Part model, mm, in its own coordinate system. Face numbers are marked on the shaded views. Round coordinates to 2 decimals unless told otherwise and drop trailing zeros. Loops run counter-clockwise (first coordinate to the right, second up) from the corner with the lowest first, then second, coordinate; pieces in that order, holes last. Notation, with made-up numbers: M -32.75,-13 L -15.75,-13 A32 cw -15.75,14 Z; hole C 62,63 d11. An arc over 180 degrees is marked long. Put each result on its own line as item: value. Start each with the question number.
1) Slice it at C-C on z = 5. Give the cut face in (x, y).
2) Probe line 1 along X through (y, z) = (21, 60); line 2 along X through (y, z) = (19, 41); line 3 along Y through (x, z) = (21, 47). List the from-to ranges inside material, lowest first.
3) Pull direction Y, two halves, no side cores. Call the marked faces 1, 2 and 3: +Y half, -Y half, draft (parallel to the pull), parting line (faces both ways), or undercut.
4) Drop flat-ended pins along their axis: pin 1 Ø1.1 at (x, y) = (2.5, 2) entering from -Z; pin 2 Ø8 at (x, z) = (27.5, 37) entering from -Y; pin 3 Ø2 at (x, z) = (21.5, 46.5) entering from +Y; pin 4 Ø0.8 at (x, z) = (30.5, 89.5) entering from -Y. Give the stop position or say it passes through.
5) Slice it at A-A on y = 5. Give the cut face in (x, z).
6) Slice it at B-B on z = 50. Give the cut face in (x, y), then the cut area to 3 significant figures.
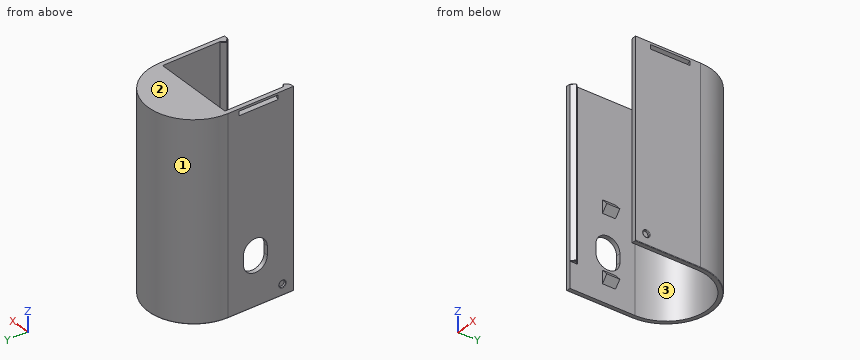
```python
from build123d import *

# Parameters (mm, degrees)
BOSS_EXTRUDE1_DEPTH = 90
BOSS_EXTRUDE2_START = -1
BOSS_EXTRUDE2_DEPTH = 1
CUT_EXTRUDE2_DEPTH  = 2
SKETCH6_R           = 1.5
CUT_EXTRUDE3_DEPTH  = 1
CUT_EXTRUDE4_DEPTH  = 18
BOSS_EXTRUDE3_DEPTH = 78
BOSS_EXTRUDE4_START = -8
BOSS_EXTRUDE4_DEPTH = 6
FILLET2_R           = 0.25
CHAMFER1_SIZE       = 0.25
FILLET3_R           = 0.25
CHAMFER2_SIZE       = 0.25


with BuildPart() as part:
    # Sketch2 → Boss-Extrude1 (new body)
    with BuildSketch(Plane.XY):
        with BuildLine():
            Line((0, 0), (0, 30))
            ThreePointArc((0, 30), (21, 51), (42, 30))
            Line((42, 30), (42, 0))
            Line((42, 0), (40, 0))
            Line((40, 0), (40, 30))
            ThreePointArc((40, 30), (21, 49), (2, 30))
            Line((2, 30), (2, 0))
            Line((2, 0), (0, 0))
        make_face()
    extrude(amount=BOSS_EXTRUDE1_DEPTH)

    # Sketch3 → Boss-Extrude2 (add)
    with BuildSketch(Plane.XY.offset(90).offset(BOSS_EXTRUDE2_START)):
        with BuildLine():
            Line((2, 30), (40, 30))
            ThreePointArc((40, 30), (21, 49), (2, 30))
        make_face()
    extrude(amount=BOSS_EXTRUDE2_DEPTH)

    # Sketch5 → Cut-Extrude2 (cut)
    with BuildSketch(Plane.ZY):
        with BuildLine():
            Line((20.5, 23), (24.5, 23))
            ThreePointArc((24.5, 23), (30, 17.5), (24.5, 12))
            Line((24.5, 12), (20.5, 12))
            ThreePointArc((20.5, 12), (15, 17.5), (20.5, 23))
        make_face()
    extrude(amount=-CUT_EXTRUDE2_DEPTH, mode=Mode.SUBTRACT)

    # Sketch6 → Cut-Extrude3 (cut)
    with BuildSketch(Plane.ZY):
        with Locations((5, 5)):
            Circle(SKETCH6_R)
    cut_extrude3 = extrude(amount=-CUT_EXTRUDE3_DEPTH, mode=Mode.SUBTRACT)

    # Mirror1: Cut-Extrude3 across plane
    add(cut_extrude3.mirror(Plane(origin=(21, 0, 0), x_dir=(0, 0, 1), z_dir=(1, 0, 0))), mode=Mode.SUBTRACT)

    # Sketch7 → Cut-Extrude4 (cut)
    with BuildSketch(Plane(origin=(0, 7, 0), x_dir=(-1, 0, 0), z_dir=(0, -1, 0))):
        Polygon((0, -89), (0, -87), (-1.732050808, -88), align=None)
    cut_extrude4 = extrude(amount=-CUT_EXTRUDE4_DEPTH, mode=Mode.SUBTRACT)

    # Mirror2: Cut-Extrude4 across plane
    add(cut_extrude4.mirror(Plane(origin=(21, 0, 0), x_dir=(0, 0, 1), z_dir=(1, 0, 0))), mode=Mode.SUBTRACT)

    # Sketch8 → Boss-Extrude3 (add)
    with BuildSketch(Plane.XY.offset(90)):
        Polygon((2, 0), (3.767766953, 1.767766953), (2, 3.535533906), align=None)
    boss_extrude3 = extrude(amount=-BOSS_EXTRUDE3_DEPTH)

    # Mirror3: Boss-Extrude3 across plane
    add(boss_extrude3.mirror(Plane(origin=(21, 0, 0), x_dir=(0, 0, 1), z_dir=(1, 0, 0))))

    # Sketch9 → Boss-Extrude4 (add)
    with BuildSketch(Plane(origin=(0, 7, 0), x_dir=(-1, 0, 0), z_dir=(0, -1, 0)).offset(BOSS_EXTRUDE4_START)):
        Polygon((-2, -8), (-2, -14), (-4.645751311, -11), align=None)
        Polygon((-2, -39), (-2, -45), (-4.645751311, -42), align=None)
    extrude(amount=-BOSS_EXTRUDE4_DEPTH)

    # Fillet2
    fillet2_edges = [part.edges().sort_by_distance(p)[0] for p in [
        (0, 5, 3.5),
        (42, 5, 3.5),
    ]]
    fillet(fillet2_edges, radius=FILLET2_R)

    # Chamfer1
    chamfer1_edges = [part.edges().sort_by_distance(p)[0] for p in [
        (2.883883476, 2.651650429, 12),
        (2.883883476, 2.651650429, 90),
        (2.883883476, 0.883883476, 90),
        (39.116116524, 2.651650429, 90),
        (39.116116524, 0.883883476, 90),
        (39.116116524, 2.651650429, 12),
    ]]
    chamfer(chamfer1_edges, length=CHAMFER1_SIZE)

    # Fillet3
    fillet3_edges = [part.edges().sort_by_distance(p)[0] for p in [
        (0, 15, 0),
        (21, 51, 0),
        (42, 15, 0),
    ]]
    fillet(fillet3_edges, radius=FILLET3_R)

    # Chamfer2
    chamfer2_edges = [part.edges().sort_by_distance(p)[0] for p in [
        (2.795495129, 0.795495129, 12),
        (39.204504871, 0.795495129, 12),
    ]]
    chamfer(chamfer2_edges, length=CHAMFER2_SIZE)


solid = part.part
```
Recorded:
1. outline: M 0,0 L 2,0 L 2,30 A19 cw 40,30 L 40,0 L 42,0 L 42,3.25 A0.25 ccw 41.75,3.5 L 41,3.5 L 41,6.5 L 41.75,6.5 A0.25 ccw 42,6.75 L 42,30 A21 ccw 0,30 L 0,6.75 A0.25 ccw 0.25,6.5 L 1,6.5 L 1,3.5 L 0.25,3.5 A0.25 ccw 0,3.25 Z
2. line 1: x = 0 to 2, 40 to 42
2. line 2: x = 0 to 3.76, 40 to 42
2. line 3: y = 49 to 51
3. face 1: +Y half
3. face 2: draft
3. face 3: undercut
4. pin 1: stops at z = 0
4. pin 2: stops at y = 45.84
4. pin 3: stops at y = 51
4. pin 4: stops at y = 30
5. outline: M 0,0.25 A0.25 ccw 0.25,0 L 2,0 L 2,90 L 0,90 L 0,6.75 A0.25 ccw 0.25,6.5 L 1,6.5 L 1,3.5 L 0.25,3.5 A0.25 ccw 0,3.25 Z; M 40,0 L 41.75,0 A0.25 ccw 42,0.25 L 42,3.25 A0.25 ccw 41.75,3.5 L 41,3.5 L 41,6.5 L 41.75,6.5 A0.25 ccw 42,6.75 L 42,90 L 40,90 Z
6. outline: M 0,0 L 2,0 L 3.77,1.77 L 2,3.54 L 2,30 A19 cw 40,30 L 40,3.54 L 38.23,1.77 L 40,0 L 42,0 L 42,30 A21 ccw 0,30 Z
6. area: 252 mm2
